Job drawing, mm, ordinate dimensions from the low corner. One solid piece. Coordinates: 2 decimals unless noted, no trailing zeros. Write each loop counter-clockwise with the first axis right and the second up, starting at its lowest first coordinate (ties: lowest second). Pieces come first, ordered by that corner, then holes. Notation, with made-up numbers: (23.5, 22.25) - (80.5, 22.25) arc R36 ccw to (80.5, 56.25) - close; hole circle Ø3 at (57, -28). An arc over 180 degrees is marked (long way). Use a Markdown table: item, result.
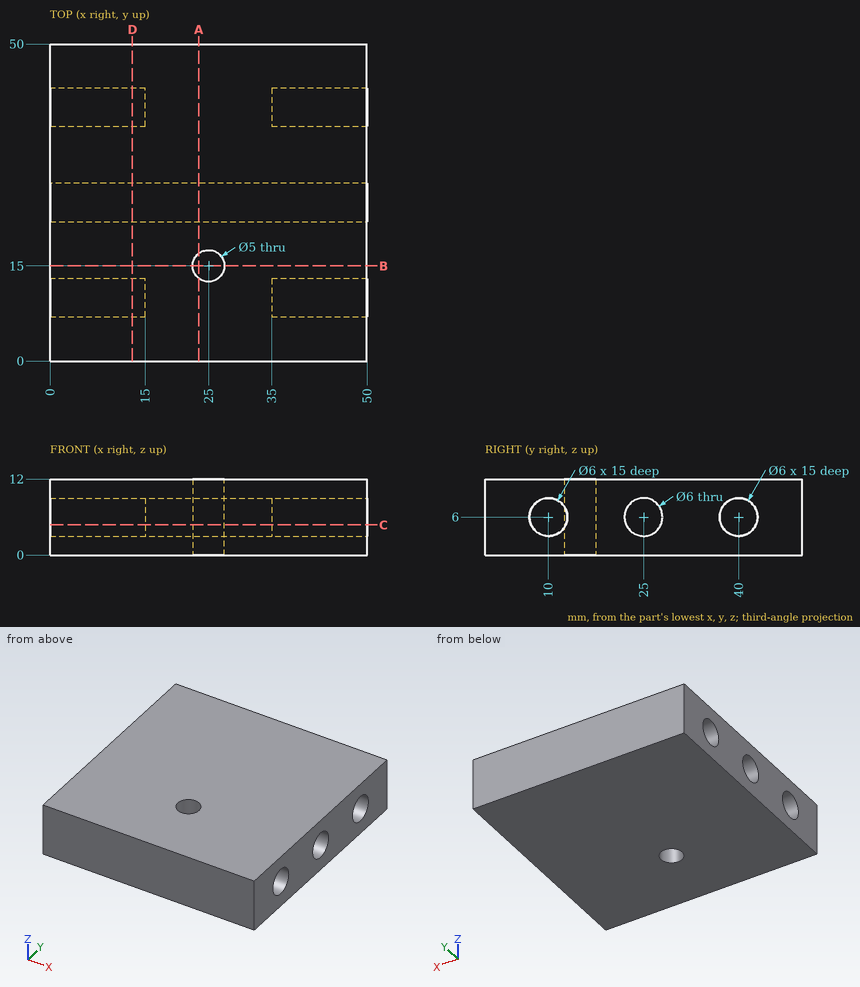
Item 1: Band-saw the part on D-D, the plane x = 13. Give the cut face in (y, z), then the cut area to 3 significant figures.
From the geometry:
| item | result |
|---|---|
| outline | (0, 0) - (50, 0) - (50, 12) - (0, 12) - close; hole circle Ø6 at (10, 6); hole circle Ø6 at (25, 6); hole circle Ø6 at (40, 6) |
| area | 515 mm^2 |
Item 2: Band-saw the part on B-B, the plane y = 15. Give the cut face in (x, z), then the cut area to 3 significant figures.
From the geometry:
| item | result |
|---|---|
| outline | (0, 0) - (22.5, 0) - (22.5, 12) - (0, 12) - close; (27.5, 0) - (50, 0) - (50, 12) - (27.5, 12) - close |
| area | 540 mm^2 |
Item 3: Band-saw the part on A-A, the plane x = 23.5. Give the cut face in (y, z).
From the geometry:
| item | result |
|---|---|
| outline | (0, 0) - (13, 0) - (13, 12) - (0, 12) - close; (17, 0) - (50, 0) - (50, 12) - (17, 12) - close; hole circle Ø6 at (25, 6) |
Item 4: Drill centre lines: probe 1 along Y at (x, z) = (25, 9.5); probe 2 along Y at (x, z) = (25, 5.75); probe 3 along Z at (x, y) = (45, 40). Where is each one in solid material? Low to high.
From the geometry:
| item | result |
|---|---|
| probe 1 | 0 to 12.5, 17.5 to 50 |
| probe 2 | 0 to 12.5, 17.5 to 22.01, 27.99 to 50 |
| probe 3 | 0 to 3, 9 to 12 |
Item 5: Drop flat-ended pins along their axis: P1, Ø3, axis at y = 40.5, z = 6, coming from the -X side; P2, Ø3, axis at y = 39.5, z = 5, coming from the +X side; P3, Ø4, axis at x = 25, y = 15, coming from the +Z side. Give the stop position or say it passes through.
From the geometry:
| item | result |
|---|---|
| P1 | x = 15 |
| P2 | x = 35 |
| P3 | through |
Item 6: Band-saw the part on C-C, the plane z = 4.75. Give the cut face in (x, y).
From the geometry:
| item | result |
|---|---|
| outline | (0, 0) - (50, 0) - (50, 7.27) - (35, 7.27) - (35, 12.73) - (50, 12.73) - (50, 22.27) - (0, 22.27) - (0, 12.73) - (15, 12.73) - (15, 7.27) - (0, 7.27) - close; (0, 27.73) - (50, 27.73) - (50, 37.27) - (35, 37.27) - (35, 42.73) - (50, 42.73) - (50, 50) - (0, 50) - (0, 42.73) - (15, 42.73) - (15, 37.27) - (0, 37.27) - close; hole circle Ø5 at (25, 15) |
